```python
from build123d import *

# Parameters (mm, degrees)
SKETCH5_W                = 120
SKETCH5_H                = 20
BOSS_EXTRUDE1_DEPTH      = 20
BOSS_EXTRUDE2_DEPTH      = 0.2
BOSS_EXTRUDE2_DEPTH_BACK = 20.2
SKETCH7_R                = 2.5
CUT_EXTRUDE1_DEPTH       = 124.320882254
BODY_MOVE_COPY1_ANGLE    = 90


with BuildPart() as part:
    # Sketch5 → Boss-Extrude1 (new body)
    with BuildSketch(Plane.XY):
        with Locations((60, 10)):
            Rectangle(SKETCH5_W, SKETCH5_H)
    extrude(amount=BOSS_EXTRUDE1_DEPTH)

    # Sketch7 → Boss-Extrude2 (add, two sides: drawn at the far end of the back side and taken through both)
    with BuildSketch(Plane(origin=(0, 20, 0), x_dir=(1, 0, 0), z_dir=(0, 1, 0)).offset(-BOSS_EXTRUDE2_DEPTH_BACK)):
        with Locations(Location((110, -10, 0), (0, 0, 270))):
            Circle(SKETCH7_R)
    extrude(amount=BOSS_EXTRUDE2_DEPTH + BOSS_EXTRUDE2_DEPTH_BACK)

    # Sketch6 → Cut-Extrude1 (cut, through all)
    with BuildSketch(Plane.XY.offset(20)):
        with BuildLine():
            Line((54.505553499, 4), (60.279056191, 14))
            ThreePointArc((60.279056191, 14), (60.279056191, 16), (58.547005384, 17))
            Line((58.547005384, 17), (47, 17))
            ThreePointArc((47, 17), (45.267949192, 16), (45.267949192, 14))
            Line((45.267949192, 14), (51.041451884, 4))
            ThreePointArc((51.041451884, 4), (52.773502692, 3), (54.505553499, 4))
        make_face()
        with BuildLine():
            Line((5, 3), (16.547005384, 3))
            ThreePointArc((16.547005384, 3), (18.279056191, 4), (18.279056191, 6))
            Line((18.279056191, 6), (12.505553499, 16))
            ThreePointArc((12.505553499, 16), (10.773502692, 17), (9.041451884, 16))
            Line((9.041451884, 16), (3.267949192, 6))
            ThreePointArc((3.267949192, 6), (3.267949192, 4), (5, 3))
        make_face()
        with BuildLine():
            Line((26.505553499, 4), (32.279056191, 14))
            ThreePointArc((32.279056191, 14), (32.279056191, 16), (30.547005384, 17))
            Line((30.547005384, 17), (19, 17))
            ThreePointArc((19, 17), (17.267949192, 16), (17.267949192, 14))
            Line((17.267949192, 14), (23.041451884, 4))
            ThreePointArc((23.041451884, 4), (24.773502692, 3), (26.505553499, 4))
        make_face()
        with BuildLine():
            Line((37.041451884, 16), (31.267949192, 6))
            ThreePointArc((31.267949192, 6), (31.267949192, 4), (33, 3))
            Line((33, 3), (44.547005384, 3))
            ThreePointArc((44.547005384, 3), (46.279056191, 4), (46.279056191, 6))
            Line((46.279056191, 6), (40.505553499, 16))
            ThreePointArc((40.505553499, 16), (38.773502692, 17), (37.041451884, 16))
        make_face()
        with BuildLine():
            Line((65.041451884, 16), (59.267949192, 6))
            ThreePointArc((59.267949192, 6), (59.267949192, 4), (61, 3))
            Line((61, 3), (72.547005384, 3))
            ThreePointArc((72.547005384, 3), (74.279056191, 4), (74.279056191, 6))
            Line((74.279056191, 6), (68.505553499, 16))
            ThreePointArc((68.505553499, 16), (66.773502692, 17), (65.041451884, 16))
        make_face()
        with BuildLine():
            Line((93.041451884, 16), (87.267949192, 6))
            ThreePointArc((87.267949192, 6), (87.267949192, 4), (89, 3))
            Line((89, 3), (100.547005384, 3))
            ThreePointArc((100.547005384, 3), (102.279056191, 4), (102.279056191, 6))
            Line((102.279056191, 6), (96.505553499, 16))
            ThreePointArc((96.505553499, 16), (94.773502692, 17), (93.041451884, 16))
        make_face()
        with BuildLine():
            Line((82.505553499, 4), (88.279056191, 14))
            ThreePointArc((88.279056191, 14), (88.279056191, 16), (86.547005384, 17))
            Line((86.547005384, 17), (75, 17))
            ThreePointArc((75, 17), (73.267949192, 16), (73.267949192, 14))
            Line((73.267949192, 14), (79.041451884, 4))
            ThreePointArc((79.041451884, 4), (80.773502692, 3), (82.505553499, 4))
        make_face()
    extrude(amount=-CUT_EXTRUDE1_DEPTH, mode=Mode.SUBTRACT)


with BuildPart() as part_1:
    # Body-Move/Copy1: moved
    add(part.part.rotate(Axis((0, 7.5, 7.5), (1, 0, 0)), BODY_MOVE_COPY1_ANGLE))


solid = part_1.part
```
CAD build for the part. Positions are in the model's coordinates, mm. A direction names the side the tool comes from. Coordinates: 2 decimals unless noted, no trailing zeros. Order: outer loops, then holes, each group sorted by start corner. A loop starts at its lowest first (then second) coordinate and runs counter-clockwise, first axis right, second up. Notation, with made-up numbers: M -25,-24.75 L 17,-24.75 A19 cw 17,-13.75 Z; hole C 18,19 d5. An arc over 180 degrees is marked long. Write each question's results on one line, items separated by ' | '. Start each with the question number.
Q1. Cut at B-B (x = 43.5). List the corners of the cut face in (y, z).
Q2. Drill centre lines: probe 1 along Z at (x, y) = (21, 6.75); probe 2 along Z at (x, y) = (16.5, 2); probe 3 along Z at (x, y) = (31.5, -3.5). Where is each one in solid material? Low to high. Write a range as from..to.
Q3. Pull direction X, two halves, no side cores. Call faces 1 (the flat face through (120, 5, 10)), 2 (the flat face through (90.195, 4.86, 11.07)), 3 (the flat face through (59, 15, 10)): +X half, -X half, draft (parallel to the pull), parting line (faces both ways), or undercut.
Q4. Cut at A-A (z = 9.75). Count the separate pieces of the cut face and the enclosed holes in it, then the cut area to 3 significant figures.
Q5. Which spindle directions (+Z, -Z, +X, -X, +Y, -Y) get a long thin tool onto all of the face, cutting with end or side? Do faces 4 (the flat face through (110, 5, 20.2)), 5 (the flat face through (34.195, 4.86, 11.07)). Say none if no direction does.
Q6. Flat gauge pins, fed straight in: P1, Ø6, axis at x = 18, y = 12, coming from the +Z side; P2, Ø1, axis at x = 61, y = 4.5, coming from the -Z side. Where does each tip first touch, or does it go through?
Found:
1) outline: M -5,0 L 15,0 L 15,3 L -5,3 Z; M -5,10.81 L 15,10.81 L 15,20 L -5,20 Z
2) probe 1: 0..7.54, 17..20 | probe 2: 0..3, 9.08..20 | probe 3: 0..3.68, 6.4..12.65, 16.76..20
3) face 1: +X half | face 2: undercut | face 3: draft
4) separate pieces: 8 | enclosed holes: 0 | area: 939 mm²
5) face 4: +Z, +X, -X, +Y, -Y | face 5: +Y, -Y
6) P1: z = 20 | P2: z = 0
